Verification items for the finished model (mm, model axes). Face numbers are marked on the shaded views. A direction names the side the tool comes from. Round coordinates to 2 decimals unless told otherwise and drop trailing zeros. Write each loop counter-clockwise with the first axis right and the second up, starting at its lowest first coordinate (ties: lowest second). Pieces come first, ordered by that corner, then holes. Notation, with made-up numbers: M -3.5,74 L 47.5,74 A20 cw 47.5,103 Z; hole C 37.5,-26 d7. An arc over 180 degrees is marked long. One line per item, written item: value. Start each with the question number.
from build123d import *

# Parameters (mm, degrees)
BOSS_EXTRUDE1_DEPTH  = 4.75
M2_CLEARANCE_HOLE1_D = 2.4
SKETCH4_R            = 2
CUT_EXTRUDE1_DEPTH   = 1.2
SKETCH5_W            = 10
SKETCH5_H            = 15
BOSS_EXTRUDE2_DEPTH  = 2
CUT_EXTRUDE2_DEPTH   = 2


with BuildPart() as part:
    # Sketch1 → Boss-Extrude1 (new, symmetric)
    with BuildSketch(Plane.XY):
        Polygon((-17.53737418, 15.5), (-17.53737418, 25.5), (-16.53737418, 25.5), (-16.53737418, 27.5), (-19.53737418, 27.5), (-19.53737418, 0), (-19.53737418, -8.11), (-11.42737418, -8.11), (3.46262582, -8.11), (3.46262582, -6.11), (-12.42737418, -6.11), (-16.53737418, -6.11), (-16.53737418, 12.5), (-16.53737418, 15.5), align=None)
    extrude(amount=BOSS_EXTRUDE1_DEPTH, both=True)

    # M2 Clearance Hole1 (through all)
    with Locations(Plane(origin=(-17.53737418, 22, 2.5), x_dir=(0, 1, 0), z_dir=(1, 0, 0))):
        with Locations((0, 0), (0, -5)):
            Hole(M2_CLEARANCE_HOLE1_D / 2)

    # Sketch4 → Cut-Extrude1 (cut)
    with BuildSketch(Plane(origin=(-17.53737418, 0, 0), x_dir=(0, 0, -1), z_dir=(1, 0, 0))):
        with Locations((-2.5, 22)):
            Circle(SKETCH4_R)
        with Locations((2.5, 22)):
            Circle(SKETCH4_R)
    extrude(amount=-CUT_EXTRUDE1_DEPTH, mode=Mode.SUBTRACT)

    # Sketch5 → Boss-Extrude2 (add)
    with BuildSketch(Plane.XZ.offset(8.11)):
        with Locations((-1.53737418, 0)):
            Rectangle(SKETCH5_W, SKETCH5_H)
    extrude(amount=-BOSS_EXTRUDE2_DEPTH)

    # Sketch6 → Cut-Extrude2 (cut)
    with BuildSketch(Plane(origin=(0, -6.11, 0), x_dir=(1, 0, 0), z_dir=(0, 1, 0))):
        with BuildLine():
            Line((-0.28737418, -5), (-2.78737418, -5))
            ThreePointArc((-2.78737418, -5), (-3.78737418, -4), (-2.78737418, -3))
            Line((-2.78737418, -3), (-0.28737418, -3))
            ThreePointArc((-0.28737418, -3), (0.71262582, -4), (-0.28737418, -5))
        make_face()
        with BuildLine():
            Line((-0.28737418, 5), (-2.78737418, 5))
            ThreePointArc((-2.78737418, 5), (-3.78737418, 4), (-2.78737418, 3))
            Line((-2.78737418, 3), (-0.28737418, 3))
            ThreePointArc((-0.28737418, 3), (0.71262582, 4), (-0.28737418, 5))
        make_face()
    extrude(amount=-CUT_EXTRUDE2_DEPTH, mode=Mode.SUBTRACT)


solid = part.part
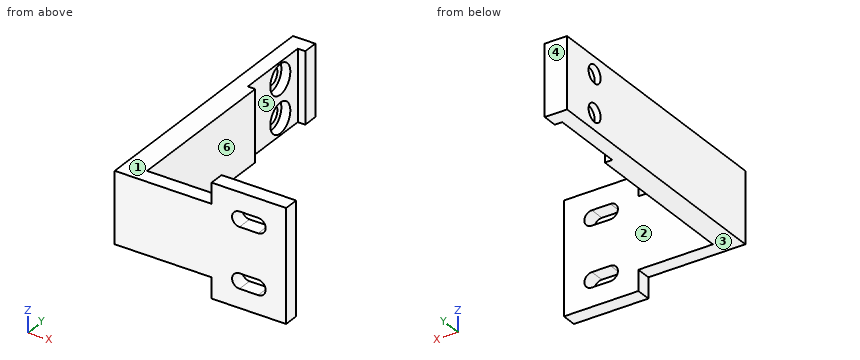
1) Cross-section at B-B (z = -2.5). Record the boundary of the cut face in (x, y).
2) Cross-section at D-D (z = -5.75). Record the boundary of the cut face in (x, y), then the cut area to 3 significant figures.
3) Gauge pin test, flat ends, axial feed: pin 1 Ø1.6 at (y, z) = (-7.5, -6.5) entering from -X; pin 2 Ø1 at (x, z) = (-5, -1) entering from +Y; pin 3 Ø10 at (x, y) = (-8, 21.5) entering from -Z; pin 4 Ø0.6 at (y, z) = (27, -2) entering from +X. Record the tip position at first contact, or that the pin passes through.
4) Thickness scan on line 1 (Z direction, x = -18.95, y = 22); line 2 (Y direction, x = -18.15, z = -2.5); line 3 (X direction, y = 23, z = 0). Record the ranges inside material, lowest first.
5) Cross-section at A-A (x = -2). Record the boundary of the cut face in (y, z).
6) Mould release check, pull along Y, two halves, no side actions. Record for the marked faces 4, 5 and 6: pulls with the +Y half, pulls with the -Y half, needs draft (parallel to the pull), parting line crosses it, or undercut.
7) Cross-section at C-C (y = 14). Record the boundary of the cut face in (x, z), then the cut area to 3 significant figures.
8) Access from +Z, -Z, +X, -X, +Y, -Y to the whole of each face (thin tool, end or side, straight path). Record for the marked faces 1, 2 and 3.
Results below:
1. outline: M -19.54,-8.11 L 3.46,-8.11 L 3.46,-6.11 L -16.54,-6.11 L -16.54,15.5 L -17.54,15.5 L -17.54,20 L -18.74,20 L -18.74,20.8 L -19.54,20.8 Z; M -19.54,23.2 L -18.74,23.2 L -18.74,24 L -17.54,24 L -17.54,25.5 L -16.54,25.5 L -16.54,27.5 L -19.54,27.5 Z
2. outline: M -6.54,-8.11 L 3.46,-8.11 L 3.46,-6.11 L -6.54,-6.11 Z
2. area: 20.0 mm²
3. pin 1: stops at x = -6.54
3. pin 2: stops at y = -6.11
3. pin 3: passes through
3. pin 4: stops at x = -16.54
4. line 1: z = -4.75 to -3.7, -1.3 to 1.3, 3.7 to 4.75
4. line 2: y = -8.11 to 20, 24 to 27.5
4. line 3: x = -19.54 to -17.54
5. outline: M -8.11,-7.5 L -6.11,-7.5 L -6.11,-5 L -8.11,-5 Z; M -8.11,-3 L -6.11,-3 L -6.11,3 L -8.11,3 Z; M -8.11,5 L -6.11,5 L -6.11,7.5 L -8.11,7.5 Z
6. face 4: pulls with the +Y half
6. face 5: undercut
6. face 6: needs draft
7. outline: M -19.54,-4.75 L -16.54,-4.75 L -16.54,4.75 L -19.54,4.75 Z
7. area: 28.5 mm²
8. face 1: +Z, -X, +Y, -Y
8. face 2: +Z, -Z, +X, +Y
8. face 3: -Z, -X, +Y, -Y
